Read the model definition and answer for the solid it produces. Units are mm, in the model's axes. Give positions to 0.01 mm unless a question says otherwise; leave off trailing zeros. Order: outer loops, then holes, each group sorted by start corner. A loop starts at its lowest first (then second) coordinate and runs counter-clockwise, first axis right, second up. Notation, with made-up numbers: (28.5, 28) - (49.5, 28) arc R22 cw to (49.5, 64) - close; hole circle Ø8 at (-13, -33.75). An arc over 180 degrees is marked (long way). Use a Markdown table: item, result. Add a question column.
1. Consider L1, parallel to X at y = 12.45, z = -93.5; L2, parallel to X at y = 12.8, z = -137.5; L3, parallel to X at y = 12.7, z = -87.5. Determine where each line is inside the solid, lowest interval first.
2. A flat-ended cylindrical pin translates along its axis: P1, Ø20, axis at x = 20.21, z = -96.82, coming from the +Y side. Find the tip coordinate at first contact, or state that the pin passes through.
3. A cutting plane is placed at C-C on y = 12.7. State how many separate pieces and enclosed holes the cut face has, and give its area (3 significant figures).
4. A cutting plane is placed at D-D on x = -12.7. Determine the outline of the cut face in (y, z) (3 decimals), and give its area (3 significant figures).
5. A cutting plane is placed at B-B on x = -57.3. Determine the outline of the cut face in (y, z) (3 decimals), and give its area (3 significant figures).
6. A cutting plane is placed at A-A on z = -98.5. Determine the outline of the cut face in (x, y) (3 decimals).
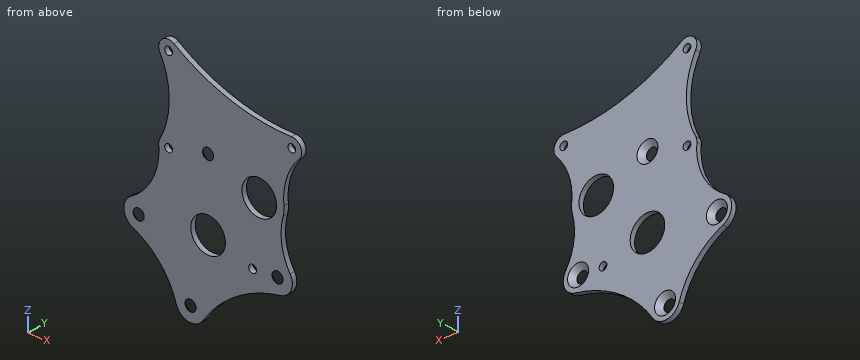
```python
from build123d import *

# Parameters (mm, degrees)
LOWEREDBALLAST_DECK_MOUNT_START       = 6.35
LOWEREDBALLAST_DECK_MOUNT_OUTLINE_R   = 2.5527
LOWEREDBALLAST_DECK_MOUNT_OUTLINE_R_2 = 2.4892
LOWEREDBALLAST_DECK_MOUNT_OUTLINE_R_3 = 8.73125
LOWEREDBALLAST_DECK_MOUNT_DEPTH       = 5.08
BODY_MOVE_COPY2_START                 = 11.43
BODY_MOVE_COPY2_OUTLINE_W             = 5.08
BODY_MOVE_COPY2_OUTLINE_H             = 241.3
BODY_MOVE_COPY2_DEPTH                 = 185.42
BODY_MOVE_COPY2_START_2               = 6.35
BODY_MOVE_COPY2_2_OUTLINE_W           = 5.08
BODY_MOVE_COPY2_2_OUTLINE_H           = 127
BODY_MOVE_COPY2_2_DEPTH               = 5.08
BODY_MOVE_COPY2_3_OUTLINE_R           = 2.5527
BODY_MOVE_COPY2_3_OUTLINE_R_2         = 2.4892
BODY_MOVE_COPY2_3_OUTLINE_R_3         = 8.73125
BODY_MOVE_COPY2_3_DEPTH               = 5.08
SKETCH2_R                             = 2.4892
SKETCH2_R_2                           = 11.1125
BOSS_EXTRUDE2_DEPTH                   = 3.175
BOSS_EXTRUDE3_DEPTH                   = 3.175
CSK_FOR_M6_SFHCS1_AT_2_COUNT          = 2
CSK_FOR_M6_SFHCS1_AT_2_PITCH          = 50.151171472
CSK_FOR_M6_SFHCS1_AT_3_COUNT          = 2
CSK_FOR_M6_SFHCS1_AT_3_PITCH          = 89.2
CSK_FOR_M6_SFHCS1_AT_4_COUNT          = 2
CSK_FOR_M6_SFHCS1_AT_4_PITCH          = 67.750719553


# Read off the part's stored shape, not the designer's step: LoweredBallast_Deck_Mount, Body-Move/Copy2
with BuildPart() as part:
    # LoweredBallast_Deck_Mount outline → LoweredBallast_Deck_Mount (new body)
    with BuildSketch(Plane.YZ.offset(LOWEREDBALLAST_DECK_MOUNT_START)):
        Polygon((6.35, -120.65), (107.712348179, -120.65), (196.85, -56.884227826), (196.85, 56.884227826), (107.712348179, 120.65), (6.35, 120.65), align=None)
        with Locations((15.875, -111.125)):
            Circle(LOWEREDBALLAST_DECK_MOUNT_OUTLINE_R, mode=Mode.SUBTRACT)
        with Locations((49.2125, -13.748153285)):
            Circle(LOWEREDBALLAST_DECK_MOUNT_OUTLINE_R, mode=Mode.SUBTRACT)
        with Locations((61.207670487, -41.07506464)):
            Circle(LOWEREDBALLAST_DECK_MOUNT_OUTLINE_R_2, mode=Mode.SUBTRACT)
        with Locations((96.823134697, -20.21447179)):
            Circle(LOWEREDBALLAST_DECK_MOUNT_OUTLINE_R_3, mode=Mode.SUBTRACT)
        with Locations((104.656174089, -111.125)):
            Circle(LOWEREDBALLAST_DECK_MOUNT_OUTLINE_R, mode=Mode.SUBTRACT)
        with Locations((137.869384338, -15.875)):
            Circle(LOWEREDBALLAST_DECK_MOUNT_OUTLINE_R_2, mode=Mode.SUBTRACT)
        with Locations((187.325, -51.986786112)):
            Circle(LOWEREDBALLAST_DECK_MOUNT_OUTLINE_R, mode=Mode.SUBTRACT)
        with Locations((15.875, 0)):
            Circle(LOWEREDBALLAST_DECK_MOUNT_OUTLINE_R, mode=Mode.SUBTRACT)
        with Locations((49.2125, 13.748153285)):
            Circle(LOWEREDBALLAST_DECK_MOUNT_OUTLINE_R, mode=Mode.SUBTRACT)
        with Locations((38.1, 38.1)):
            Circle(LOWEREDBALLAST_DECK_MOUNT_OUTLINE_R_2, mode=Mode.SUBTRACT)
        with Locations((57.15, 0)):
            Circle(LOWEREDBALLAST_DECK_MOUNT_OUTLINE_R_3, mode=Mode.SUBTRACT)
        with Locations((73.025, 0)):
            Circle(LOWEREDBALLAST_DECK_MOUNT_OUTLINE_R, mode=Mode.SUBTRACT)
        with Locations((92.075, 38.1)):
            Circle(LOWEREDBALLAST_DECK_MOUNT_OUTLINE_R_2, mode=Mode.SUBTRACT)
        with Locations((15.875, 111.125)):
            Circle(LOWEREDBALLAST_DECK_MOUNT_OUTLINE_R, mode=Mode.SUBTRACT)
        with Locations((187.325, 51.986786112)):
            Circle(LOWEREDBALLAST_DECK_MOUNT_OUTLINE_R, mode=Mode.SUBTRACT)
        with Locations((104.656174089, 111.125)):
            Circle(LOWEREDBALLAST_DECK_MOUNT_OUTLINE_R, mode=Mode.SUBTRACT)
    extrude(amount=LOWEREDBALLAST_DECK_MOUNT_DEPTH)

    # Body-Move/Copy2 outline → Body-Move/Copy2 (cut)
    with BuildSketch(Plane(origin=(0, 0, 0), x_dir=(1, 0, 0), z_dir=(0, 1, 0)).offset(BODY_MOVE_COPY2_START)):
        with Locations((8.89, 0)):
            Rectangle(BODY_MOVE_COPY2_OUTLINE_W, BODY_MOVE_COPY2_OUTLINE_H)
    extrude(amount=BODY_MOVE_COPY2_DEPTH, mode=Mode.SUBTRACT)

    # Body-Move_Copy2 2 outline → Body-Move_Copy2 2 (cut)
    with BuildSketch(Plane(origin=(0, 0, 0), x_dir=(1, 0, 0), z_dir=(0, 1, 0)).offset(BODY_MOVE_COPY2_START_2)):
        with Locations((8.89, -57.15)):
            Rectangle(BODY_MOVE_COPY2_2_OUTLINE_W, BODY_MOVE_COPY2_2_OUTLINE_H)
        with BuildLine():
            ThreePointArc((11.43, 50.281351083), (11.195453285, 49.2125), (11.43, 48.143648917))
            Line((11.43, 48.143648917), (11.43, 50.281351083))
        make_face()
        with BuildLine():
            Line((6.35, 63.142681083), (6.35, 51.157318917))
            ThreePointArc((6.35, 51.157318917), (8.73125, 57.15), (6.35, 63.142681083))
        make_face()
    extrude(amount=BODY_MOVE_COPY2_2_DEPTH, mode=Mode.SUBTRACT)

    # Body-Move_Copy2 3 outline → Body-Move_Copy2 3 (add)
    with BuildSketch(Plane(origin=(0, 0, 0), x_dir=(1, 0, 0), z_dir=(0, 1, 0)).offset(BODY_MOVE_COPY2_START_2)):
        with BuildLine():
            Line((120.65, 6.35), (120.65, 107.712348179))
            Line((120.65, 107.712348179), (56.884227826, 196.85))
            Line((56.884227826, 196.85), (-56.884227826, 196.85))
            Line((-56.884227826, 196.85), (-120.65, 107.712348179))
            Line((-120.65, 107.712348179), (-120.65, 6.35))
            Line((-120.65, 6.35), (6.35, 6.35))
            Line((6.35, 6.35), (6.35, 51.157318917))
            ThreePointArc((6.35, 51.157318917), (-8.73125, 57.15), (6.35, 63.142681083))
            Line((6.35, 63.142681083), (6.35, 120.65))
            Line((6.35, 120.65), (11.43, 120.65))
            Line((11.43, 120.65), (11.43, 50.281351083))
            ThreePointArc((11.43, 50.281351083), (16.300853285, 49.2125), (11.43, 48.143648917))
            Line((11.43, 48.143648917), (11.43, 6.35))
            Line((11.43, 6.35), (120.65, 6.35))
        make_face()
        with Locations((-111.125, 15.875)):
            Circle(BODY_MOVE_COPY2_3_OUTLINE_R, mode=Mode.SUBTRACT)
        with Locations((0, 15.875)):
            Circle(BODY_MOVE_COPY2_3_OUTLINE_R, mode=Mode.SUBTRACT)
        with Locations((111.125, 15.875)):
            Circle(BODY_MOVE_COPY2_3_OUTLINE_R, mode=Mode.SUBTRACT)
        with Locations((-111.125, 104.656174089)):
            Circle(BODY_MOVE_COPY2_3_OUTLINE_R, mode=Mode.SUBTRACT)
        with Locations((-38.1, 38.1)):
            Circle(BODY_MOVE_COPY2_3_OUTLINE_R_2, mode=Mode.SUBTRACT)
        with Locations((-13.748153285, 49.2125)):
            Circle(BODY_MOVE_COPY2_3_OUTLINE_R, mode=Mode.SUBTRACT)
        with Locations((-38.1, 92.075)):
            Circle(BODY_MOVE_COPY2_3_OUTLINE_R_2, mode=Mode.SUBTRACT)
        with Locations((-51.986786112, 187.325)):
            Circle(BODY_MOVE_COPY2_3_OUTLINE_R, mode=Mode.SUBTRACT)
        with Locations((0, 73.025)):
            Circle(BODY_MOVE_COPY2_3_OUTLINE_R, mode=Mode.SUBTRACT)
        with Locations((41.07506464, 61.207670487)):
            Circle(BODY_MOVE_COPY2_3_OUTLINE_R_2, mode=Mode.SUBTRACT)
        with Locations((20.21447179, 96.823134697)):
            Circle(BODY_MOVE_COPY2_3_OUTLINE_R_3, mode=Mode.SUBTRACT)
        with Locations((111.125, 104.656174089)):
            Circle(BODY_MOVE_COPY2_3_OUTLINE_R, mode=Mode.SUBTRACT)
        with Locations((15.875, 137.869384338)):
            Circle(BODY_MOVE_COPY2_3_OUTLINE_R_2, mode=Mode.SUBTRACT)
        with Locations((51.986786112, 187.325)):
            Circle(BODY_MOVE_COPY2_3_OUTLINE_R, mode=Mode.SUBTRACT)
    extrude(amount=BODY_MOVE_COPY2_3_DEPTH)


with BuildPart() as body_2:
    # Sketch2 → Boss-Extrude2 (new body)
    with BuildSketch(Plane(origin=(0, 11.43, 0), x_dir=(1, 0, 0), z_dir=(0, 1, 0))):
        with BuildLine():
            ThreePointArc((-43.697395055, 41.098611111), (-42.344618776, 33.377107725), (-34.523029987, 32.853307182))
            ThreePointArc((-34.523029987, 32.853307182), (1.435165075, 49.833263975), (40.88179348, 54.860612408))
            ThreePointArc((40.88179348, 54.860612408), (46.845610099, 58.557518585), (45.763526107, 65.490289905))
            ThreePointArc((45.763526107, 65.490289905), (37.701905828, 79.281344599), (36.002655059, 95.16515579))
            ThreePointArc((36.002655059, 95.16515579), (35.295571353, 101.780559529), (31.939672665, 107.525250816))
            ThreePointArc((31.939672665, 107.525250816), (23.883267234, 121.31935255), (22.19002211, 137.203805076))
            ThreePointArc((22.19002211, 137.203805076), (20.070189732, 142.636236875), (14.412445618, 144.048658946))
            ThreePointArc((14.412445618, 144.048658946), (3.462344959, 143.086426048), (-7.306729609, 145.290429122))
            ThreePointArc((-7.306729609, 145.290429122), (-22.309274144, 142.996002148), (-28.529000968, 129.152023822))
            ThreePointArc((-28.529000968, 129.152023822), (-31.43370737, 111.399097034), (-42.15980047, 96.957675511))
            ThreePointArc((-42.15980047, 96.957675511), (-44.332497578, 93.290925139), (-43.697395055, 89.076388889))
            ThreePointArc((-43.697395055, 89.076388889), (-37.676555497, 65.0875), (-43.697395055, 41.098611111))
        make_face()
        with Locations(Location((-38.1, 92.075, 0), (0, 0, 270))):
            Circle(SKETCH2_R, mode=Mode.SUBTRACT)
        with Locations(Location((15.875, 137.869384338, 0), (0, 0, 270))):
            Circle(SKETCH2_R, mode=Mode.SUBTRACT)
        with Locations(Location((41.07506464, 61.207670487, 0), (0, 0, 270))):
            Circle(SKETCH2_R, mode=Mode.SUBTRACT)
        with Locations(Location((20.21447179, 96.823134697, 0), (0, 0, 270))):
            Circle(SKETCH2_R_2, mode=Mode.SUBTRACT)
        with Locations(Location((-12.7, 130.359646842, 0), (0, 0, 270))):
            Circle(SKETCH2_R_2, mode=Mode.SUBTRACT)
        with Locations(Location((-38.1, 38.1, 0), (0, 0, 270))):
            Circle(SKETCH2_R, mode=Mode.SUBTRACT)
    extrude(amount=BOSS_EXTRUDE2_DEPTH)

    # Sketch5 → Boss-Extrude3 (add)
    with BuildSketch(Plane(origin=(0, 14.605, 0), x_dir=(1, 0, 0), z_dir=(0, 1, 0))):
        with BuildLine():
            ThreePointArc((-61.148803131, 145.072415601), (-66.802064537, 137.020248494), (-62.317406726, 128.263273904))
            ThreePointArc((-62.317406726, 128.263273904), (-48.335449579, 112.968704409), (-44.42671909, 92.618254593))
            ThreePointArc((-44.42671909, 92.618254593), (-43.728284874, 95.015222675), (-42.15980047, 96.957675511))
            ThreePointArc((-42.15980047, 96.957675511), (-31.43370737, 111.399097034), (-28.529000968, 129.152023822))
            ThreePointArc((-28.529000968, 129.152023822), (-22.309274144, 142.996002148), (-7.306729609, 145.290429122))
            ThreePointArc((-7.306729609, 145.290429122), (3.462344959, 143.086426048), (14.412445618, 144.048658946))
            ThreePointArc((14.412445618, 144.048658946), (20.070189732, 142.636236875), (22.19002211, 137.203805076))
            ThreePointArc((22.19002211, 137.203805076), (23.883267234, 121.31935255), (31.939672665, 107.525250816))
            ThreePointArc((31.939672665, 107.525250816), (34.118030208, 104.485163692), (35.524712446, 101.019818631))
            ThreePointArc((35.524712446, 101.019818631), (34.573862159, 116.629433393), (39.973858004, 131.306089488))
            ThreePointArc((39.973858004, 131.306089488), (40.627735004, 140.174390174), (33.674724287, 145.71785066))
            ThreePointArc((33.674724287, 145.71785066), (5.421674261, 157.303422607), (-16.014164602, 179.051183993))
            ThreePointArc((-16.014164602, 179.051183993), (-25.324336968, 183.292130958), (-33.106697868, 176.65136297))
            ThreePointArc((-33.106697868, 176.65136297), (-43.690598599, 157.809698398), (-61.148803131, 145.072415601))
        make_face()
    extrude(amount=-BOSS_EXTRUDE3_DEPTH)

    # Sketch7 → CSK for M6 SFHCS1 (revolve, cut)
    with BuildSketch(Plane(origin=(-57.3, 14.605, -136.359646842), x_dir=(0, 0, 1), z_dir=(1, 0, 0))):
        Polygon((0, 0), (0, 3.175), (3.3, 3.175), (3.3, 3.42), (6.72, 0), align=None)
    csk_for_m6_sfhcs1 = revolve(axis=Axis((-57.3, 20.955, -136.359646842), (0, -1, 0)), mode=Mode.SUBTRACT)

    # CSK for M6 SFHCS1 at 2: CSK for M6 SFHCS1 ×2
    with Locations(*[Vector(0.663992465633312, -2.603373438029753e-15, -0.7477392631005777) * (i * CSK_FOR_M6_SFHCS1_AT_2_PITCH) for i in range(1, CSK_FOR_M6_SFHCS1_AT_2_COUNT)]):
        add(csk_for_m6_sfhcs1, mode=Mode.SUBTRACT)

    # CSK for M6 SFHCS1 at 3: CSK for M6 SFHCS1 ×2
    with Locations(*[(i * CSK_FOR_M6_SFHCS1_AT_3_PITCH, 0, 0) for i in range(1, CSK_FOR_M6_SFHCS1_AT_3_COUNT)]):
        add(csk_for_m6_sfhcs1, mode=Mode.SUBTRACT)

    # CSK for M6 SFHCS1 at 4: CSK for M6 SFHCS1 ×2
    with Locations(*[Vector(0.6582955914566169, 2.6219010677824987e-15, 0.7527595328315564) * (i * CSK_FOR_M6_SFHCS1_AT_4_PITCH) for i in range(1, CSK_FOR_M6_SFHCS1_AT_4_COUNT)]):
        add(csk_for_m6_sfhcs1, mode=Mode.SUBTRACT)


solid = body_2.part
```
Output values:
| question | item | result |
|---|---|---|
| 1 | L1 | -44.36 to -40.14, -36.06 to 9.61, 30.82 to 35.86 |
| 1 | L2 | -66.76 to -62.08, -52.52 to -21.21, -4.19 to 13.41, 18.34 to 27.12, 36.68 to 41.36 |
| 1 | L3 | -42.89 to -17.01, -8.39 to 14.17, 26.26 to 35.97 |
| 2 | P1 | through |
| 3 | separate pieces | 1 |
| 3 | enclosed holes | 10 |
| 3 | area | 8,900 mm² |
| 4 | outline | (11.43, -174.351) - (14.605, -174.351) - (14.605, -141.472) - (11.43, -141.472) - close; (11.43, -119.247) - (14.605, -119.247) - (14.605, -92.08) - (11.43, -88.905) - close; (11.43, -81.815) - (14.605, -78.64) - (14.605, -44.784) - (11.43, -44.784) - close |
| 4 | area | 308 mm² |
| 5 | outline | (11.43, -146.971) - (14.605, -146.971) - (14.605, -143.08) - (11.43, -139.905) - close; (11.43, -132.815) - (14.605, -129.64) - (14.605, -124.553) - (11.43, -124.553) - close |
| 5 | area | 38.6 mm² |
| 6 | outline | (-44.377, 11.43) - (9.229, 11.43) - (9.229, 14.605) - (-44.377, 14.605) - close; (31.2, 11.43) - (36.001, 11.43) - (36.001, 14.605) - (31.2, 14.605) - close |
